```python
from build123d import *

# Parameters (mm, degrees)
SKETCH1_R           = 7.9375
BOSS_EXTRUDE1_DEPTH = 5.08
SKETCH2_R           = 11.303
BOSS_EXTRUDE2_DEPTH = 59.69
SKETCH3_R           = 8.001
BOSS_EXTRUDE3_DEPTH = 80.01
SKETCH4_R           = 7.6835
BOSS_EXTRUDE4_DEPTH = 80.01
SKETCH6_W           = 5.08
SKETCH6_H           = 12.7
BOSS_EXTRUDE5_DEPTH = 10.01
FILLET1_R           = 5
SKETCH7_R           = 6.35
BOSS_EXTRUDE6_DEPTH = 26.67
SKETCH8_R           = 5.588
BOSS_EXTRUDE7_DEPTH = 21.59


with BuildPart() as part:
    # Sketch1 → Boss-Extrude1 (new body)
    with BuildSketch(Plane.XY):
        Circle(SKETCH1_R)
    boss_extrude1 = extrude(amount=BOSS_EXTRUDE1_DEPTH)

    # Sketch2 → Boss-Extrude2 (add)
    with BuildSketch(Plane.XY.offset(5.08)):
        with Locations(Location((0, 0, 0), (0, 0, 180))):
            Circle(SKETCH2_R)
    boss_extrude2 = extrude(amount=BOSS_EXTRUDE2_DEPTH)

    # Sketch3 → Boss-Extrude3 (add)
    with BuildSketch(Plane.XY.offset(64.77)):
        Circle(SKETCH3_R)
    boss_extrude3 = extrude(amount=BOSS_EXTRUDE3_DEPTH)

    # Sketch4 → Boss-Extrude4 (add)
    with BuildSketch(Plane.XY.offset(144.78)):
        Circle(SKETCH4_R)
    boss_extrude4 = extrude(amount=BOSS_EXTRUDE4_DEPTH)

    # Sketch6 → Boss-Extrude5 (add)
    with BuildSketch(Plane(origin=(0, 0, 0), x_dir=(0, 0, -1), z_dir=(1, 0, 0))):
        with Locations((-69.261191794, 0)):
            Rectangle(SKETCH6_W, SKETCH6_H)
    extrude(amount=-BOSS_EXTRUDE5_DEPTH)

    # Fillet1
    fillet1_edges = [part.edges().sort_by_distance(p)[0] for p in [
        (-10.01, -6.35, 69.261191794),
        (-10.01, 6.35, 69.261191794),
    ]]
    fillet(fillet1_edges, radius=FILLET1_R)

    # Sketch7 → Boss-Extrude6 (add)
    with BuildSketch(Plane(origin=(0, 0, 0), x_dir=(0, 0, -1), z_dir=(1, 0, 0))):
        with Locations((-92.78865741, 0)):
            Circle(SKETCH7_R)
    boss_extrude6 = extrude(amount=BOSS_EXTRUDE6_DEPTH)

    # Sketch8 → Boss-Extrude7 (add)
    with BuildSketch(Plane(origin=(26.67, 0, 0), x_dir=(0, 0, -1), z_dir=(1, 0, 0))):
        with Locations((-92.78865741, 0)):
            Circle(SKETCH8_R)
    boss_extrude7 = extrude(amount=BOSS_EXTRUDE7_DEPTH)

    # Mirror2: Boss-Extrude1, Boss-Extrude2, Boss-Extrude3, Boss-Extrude4, Boss-Extrude6, Boss-Extrude7 across plane
    add(boss_extrude1.mirror(Plane(origin=(48.26, 0, 92.78865741), x_dir=(0, 0, 1), z_dir=(1, 0, 0))))
    add(boss_extrude2.mirror(Plane(origin=(48.26, 0, 92.78865741), x_dir=(0, 0, 1), z_dir=(1, 0, 0))))
    add(boss_extrude3.mirror(Plane(origin=(48.26, 0, 92.78865741), x_dir=(0, 0, 1), z_dir=(1, 0, 0))))
    add(boss_extrude4.mirror(Plane(origin=(48.26, 0, 92.78865741), x_dir=(0, 0, 1), z_dir=(1, 0, 0))))
    add(boss_extrude6.mirror(Plane(origin=(48.26, 0, 92.78865741), x_dir=(0, 0, 1), z_dir=(1, 0, 0))))
    add(boss_extrude7.mirror(Plane(origin=(48.26, 0, 92.78865741), x_dir=(0, 0, 1), z_dir=(1, 0, 0))))


solid = part.part
```
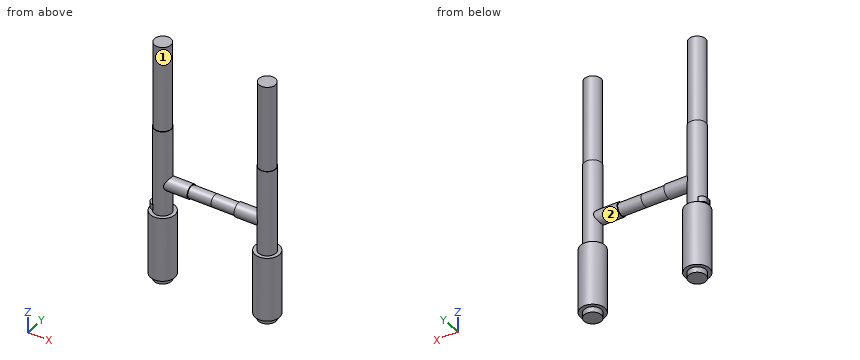
The model under review builds one solid part; all positions refer to its coordinate system, in mm. Face numbers are marked on the shaded views. A direction names the side the tool comes from. Round coordinates to 2 decimals unless told otherwise and drop trailing zeros. Write each loop counter-clockwise with the first axis right and the second up, starting at its lowest first coordinate (ties: lowest second). Pieces come first, ordered by that corner, then holes. Notation, with made-up numbers: (-14.5, -8) - (21.5, -8) arc R18 ccw to (21.5, -4) - close; hole circle Ø2 at (-7.5, 5.5). An arc over 180 degrees is marked (long way). Use one line per item in the form item = value.
Q1. For line 1 (X direction, y = -8.25, z = 11); line 2 (X direction, y = 0.5, z = 44); line 3 (Z direction, x = 23, y = -0.75), list the stretches that pass through material, from the lowest coordinate up. Write a range as [from, to].
Answer key:
line_1 = [-7.73, 7.73], [88.79, 104.25]
line_2 = [-11.29, 11.29], [85.23, 107.81]
line_3 = [86.48, 99.09]
Q2. Consider section A-A (z = 46). State the section outline as (x, y) points, and give its area (3 significant figures).
Answer key:
outline = circle Ø22.61 at (0, 0); circle Ø22.61 at (96.52, 0)
area = 803 mm2
Q3. Consider section C-C (z = 168). State the section outline as (x, y) points, and give its area (3 significant figures).
Answer key:
outline = circle Ø15.37 at (0, 0); circle Ø15.37 at (96.52, 0)
area = 371 mm2
Q4. Tool access review of the marked faces 1 and 2: name each direction out of +Z, -Z, +X, -X, +Y, -Y from which nothing blocks a thin tool from reaching the whole face with its end or side.
Answer key:
face_1 = +Z
face_2 = none
Q5. Consider section D-D (x = 58). State the section outline as (y, z) points.
Answer key:
outline = circle Ø11.18 at (0, 92.79)
Q6. Consider section B-B (x = 96.52). State the section outline as (y, z) points, and give its area (3 significant figures).
Answer key:
outline = (-11.3, 5.08) - (-7.94, 5.08) - (-7.94, 0) - (7.94, 0) - (7.94, 5.08) - (11.3, 5.08) - (11.3, 64.77) - (8, 64.77) - (8, 144.78) - (7.68, 144.78) - (7.68, 224.79) - (-7.68, 224.79) - (-7.68, 144.78) - (-8, 144.78) - (-8, 64.77) - (-11.3, 64.77) - close
area = 3,940 mm2
Q7. Insertion check: pin 1 Ø6 at (y, z) = (8, 33) entering from +X; pin 2 Ø10 at (y, z) = (1, 91.5) entering from +X; pin 3 Ø1.4 at (y, z) = (0.5, 69) entering from -X. Each pin has a flat end and moves straight along its axis. Give the tip position at first contact, or say it passes through.
Answer key:
pin_1 = 106.66
pin_2 = 104.52
pin_3 = -10.01
